Source: CAD feature listing. Evaluate the final solid. Frame: model axes, mm. Round coordinates to 2 decimals unless told otherwise and drop trailing zeros. Order: outer loops, then holes, each group sorted by start corner. A loop starts at its lowest first (then second) coordinate and runs counter-clockwise, first axis right, second up. Notation, with made-up numbers: (38.25, 50.5) - (89.25, 50.5) arc R37 ccw to (89.25, 86.5) - close; hole circle Ø2 at (40, -27.75). An arc over 180 degrees is marked (long way). Return JSON: item names as keys, results as strings. Group by question number.
1) Ray query, line 1 (Y direction, x = -19, z = 1.2); line 2 (Y direction, x = -143, z = 0.45); line 3 (Y direction, x = -332, z = 3.4). Return the intervals inside material, ascending. Write a range as from..to.
2) Section B-B, the plane y = -11. Give the number of separate pieces and of enclosed holes in the cut face, plus the area to 3 significant figures.
3) Section A-A, the plane x = -371. Return loops of the section in (y, z).
4) Section C-C, the plane x = -61.5. Return loops of the section in (y, z).
5) Mould query, pull axis Y, two halves, no side actions, for faces 1 (the cylindrical face through (-47.32, -13.43, 2.46)), 2 (the flat face through (-198, -20, 0)). Classes: pulls with the +Y half, pulls with the -Y half, needs draft (parallel to the pull), parting line crosses it, or undercut.
```python
from build123d import *

# Parameters (mm, degrees)
IZIM1_W                     = 390
IZIM1_H                     = 40
IZIM1_R                     = 4
Y_KSEKLIK_EKSTR_ZYON1_DEPTH = 5
KES_EKSTR_ZYON1_DEPTH       = 90


with BuildPart() as part:
    # Çizim1 → Yükseklik-Ekstrüzyon1 (new body)
    with BuildSketch(Plane.XY):
        with Locations((-195, -20)):
            Rectangle(IZIM1_W, IZIM1_H)
        with Locations((-371, -11)):
            Circle(IZIM1_R, mode=Mode.SUBTRACT)
        with Locations((-345.857142857, -11)):
            Circle(IZIM1_R, mode=Mode.SUBTRACT)
        with Locations((-320.714285714, -11)):
            Circle(IZIM1_R, mode=Mode.SUBTRACT)
        with Locations((-295.571428571, -11)):
            Circle(IZIM1_R, mode=Mode.SUBTRACT)
        with Locations((-270.428571429, -11)):
            Circle(IZIM1_R, mode=Mode.SUBTRACT)
        with Locations((-245.285714286, -11)):
            Circle(IZIM1_R, mode=Mode.SUBTRACT)
        with Locations((-220.142857143, -11)):
            Circle(IZIM1_R, mode=Mode.SUBTRACT)
        with Locations((-195, -11)):
            Circle(IZIM1_R, mode=Mode.SUBTRACT)
        with Locations((-169.857142857, -11)):
            Circle(IZIM1_R, mode=Mode.SUBTRACT)
        with Locations((-144.714285714, -11)):
            Circle(IZIM1_R, mode=Mode.SUBTRACT)
        with Locations((-119.571428571, -11)):
            Circle(IZIM1_R, mode=Mode.SUBTRACT)
        with Locations((-94.428571429, -11)):
            Circle(IZIM1_R, mode=Mode.SUBTRACT)
        with Locations((-69.285714286, -11)):
            Circle(IZIM1_R, mode=Mode.SUBTRACT)
        with Locations((-44.142857143, -11)):
            Circle(IZIM1_R, mode=Mode.SUBTRACT)
        with Locations((-19, -11)):
            Circle(IZIM1_R, mode=Mode.SUBTRACT)
    extrude(amount=Y_KSEKLIK_EKSTR_ZYON1_DEPTH)

    # Çizim2 → Kes-Ekstrüzyon1 (cut)
    with BuildSketch(Plane.XY.offset(5)):
        with BuildLine():
            Line((-343.395447279, -31.527866379), (-323.983252141, -31.527866379))
            ThreePointArc((-323.983252141, -31.527866379), (-321.983252141, -33.527866379), (-323.983252141, -35.527866379))
            Line((-323.983252141, -35.527866379), (-343.395447279, -35.527866379))
            ThreePointArc((-343.395447279, -35.527866379), (-345.395447279, -33.527866379), (-343.395447279, -31.527866379))
        make_face()
        with BuildLine():
            Line((-253.395447279, -31.527866379), (-233.983252141, -31.527866379))
            ThreePointArc((-233.983252141, -31.527866379), (-231.983252141, -33.527866379), (-233.983252141, -35.527866379))
            Line((-233.983252141, -35.527866379), (-253.395447279, -35.527866379))
            ThreePointArc((-253.395447279, -35.527866379), (-255.395447279, -33.527866379), (-253.395447279, -31.527866379))
        make_face()
        with BuildLine():
            Line((-163.395447279, -31.527866379), (-143.983252141, -31.527866379))
            ThreePointArc((-143.983252141, -31.527866379), (-141.983252141, -33.527866379), (-143.983252141, -35.527866379))
            Line((-143.983252141, -35.527866379), (-163.395447279, -35.527866379))
            ThreePointArc((-163.395447279, -35.527866379), (-165.395447279, -33.527866379), (-163.395447279, -31.527866379))
        make_face()
        with BuildLine():
            Line((-73.395447279, -31.527866379), (-53.983252141, -31.527866379))
            ThreePointArc((-53.983252141, -31.527866379), (-51.983252141, -33.527866379), (-53.983252141, -35.527866379))
            Line((-53.983252141, -35.527866379), (-73.395447279, -35.527866379))
            ThreePointArc((-73.395447279, -35.527866379), (-75.395447279, -33.527866379), (-73.395447279, -31.527866379))
        make_face()
    extrude(amount=-KES_EKSTR_ZYON1_DEPTH, mode=Mode.SUBTRACT)


solid = part.part
```
Geometry check:
{
 "1": {"line 1": "-40..-15, -7..0", "line 2": "-40..-35.27, -31.79..-14.61, -7.39..0", "line 3": "-40..-35.53, -31.53..0"},
 "2": {"separate pieces": "16", "enclosed holes": "0", "area": "1,350 mm2"},
 "3": {"outline": "(-40, 0) - (-15, 0) - (-15, 5) - (-40, 5) - close; (-7, 0) - (0, 0) - (0, 5) - (-7, 5) - close"},
 "4": {"outline": "(-40, 0) - (-35.53, 0) - (-35.53, 5) - (-40, 5) - close; (-31.53, 0) - (0, 0) - (0, 5) - (-31.53, 5) - close"},
 "5": {"face 1": "undercut", "face 2": "needs draft"}
}
